from build123d import *

# Parameters (mm, degrees)
SKETCH1_W           = 50.8
SKETCH1_H           = 38.1
BOSS_EXTRUDE1_DEPTH = 19.05
SKETCH2_W           = 44.45
SKETCH2_H           = 31.75
CUT_EXTRUDE1_DEPTH  = 12.7
SKETCH3_R           = 4.7625
SKETCH3_R_2         = 2.38125
CUT_EXTRUDE2_DEPTH  = 42.639734629
SKETCH4_W           = 7.9375
SKETCH4_H           = 7.9375
BOSS_EXTRUDE2_DEPTH = 12.7
SKETCH5_R           = 1.778
CUT_EXTRUDE3_DEPTH  = 42.639734629


with BuildPart() as part:
    # Sketch1 → Boss-Extrude1 (new body)
    with BuildSketch(Plane.XY):
        with Locations((6.35, 0)):
            Rectangle(SKETCH1_W, SKETCH1_H)
    extrude(amount=-BOSS_EXTRUDE1_DEPTH)

    # Sketch2 → Cut-Extrude1 (cut)
    with BuildSketch(Plane(origin=(0, 0, -19.05), x_dir=(-1, 0, 0), z_dir=(0, 0, -1))):
        with Locations((-6.35, 0)):
            Rectangle(SKETCH2_W, SKETCH2_H)
    extrude(amount=-CUT_EXTRUDE1_DEPTH, mode=Mode.SUBTRACT)

    # Sketch3 → Cut-Extrude2 (cut, through all)
    with BuildSketch(Plane.XY):
        Circle(SKETCH3_R)
        with Locations((17.462302917, 0.082964446)):
            Circle(SKETCH3_R_2)
    extrude(amount=-CUT_EXTRUDE2_DEPTH, mode=Mode.SUBTRACT)

    # Sketch4 → Boss-Extrude2 (add)
    with BuildSketch(Plane(origin=(0, 0, -6.35), x_dir=(-1, 0, 0), z_dir=(0, 0, -1))):
        with Locations((-27.78125, 15.08125)):
            Rectangle(SKETCH4_W, SKETCH4_H)
        with Locations((15.08125, 15.08125)):
            Rectangle(SKETCH4_W, SKETCH4_H)
        with Locations((15.08125, -15.08125)):
            Rectangle(SKETCH4_W, SKETCH4_H)
        with Locations((-27.78125, -15.08125)):
            Rectangle(SKETCH4_W, SKETCH4_H)
    extrude(amount=BOSS_EXTRUDE2_DEPTH)

    # Sketch5 → Cut-Extrude3 (cut, through all)
    with BuildSketch(Plane(origin=(0, 0, -19.05), x_dir=(-1, 0, 0), z_dir=(0, 0, -1))):
        with Locations((-27.78125, 15.08125)):
            Circle(SKETCH5_R)
        with Locations((15.08125, 15.08125)):
            Circle(SKETCH5_R)
        with Locations((15.08125, -15.08125)):
            Circle(SKETCH5_R)
        with Locations((-27.78125, -15.08125)):
            Circle(SKETCH5_R)
    extrude(amount=-CUT_EXTRUDE3_DEPTH, mode=Mode.SUBTRACT)


solid = part.part
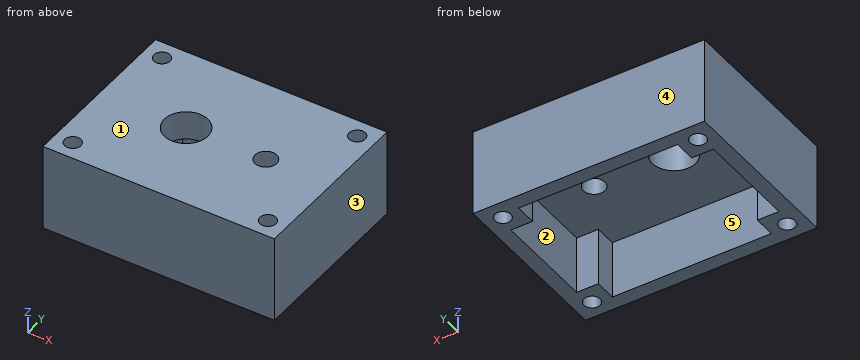
Geometry: final body of the model. Coordinates: model frame, mm. Face numbers are marked on the shaded views. A direction names the side the tool comes from. Give positions to 0.01 mm unless a question says otherwise; leave off trailing zeros. Order: outer loops, then holes, each group sorted by start corner. A loop starts at its lowest first (then second) coordinate and runs counter-clockwise, first axis right, second up. Notation, with made-up numbers: (-10, 43) -> (-6, 43) arc R36 ccw to (-6, 78) -> close; hole circle Ø9 at (81.25, -38). An arc over 180 degrees is marked (long way). Put each result on its own line as item: value.
Q1. Section C-C, the plane x = -15. Return loops of the section in (y, z).
Here are the results:
outline: (-19.05, -19.05) -> (-16.86, -19.05) -> (-16.86, 0) -> (-19.05, 0) -> close; (-13.31, -19.05) -> (-11.11, -19.05) -> (-11.11, -6.35) -> (11.11, -6.35) -> (11.11, -19.05) -> (13.31, -19.05) -> (13.31, 0) -> (-13.31, 0) -> close; (16.86, -19.05) -> (19.05, -19.05) -> (19.05, 0) -> (16.86, 0) -> close
Q2. Section B-B, the plane y = -9. Return loops of the section in (x, z) (3 decimals).
Here are the results:
outline: (-19.05, -19.05) -> (-15.875, -19.05) -> (-15.875, -6.35) -> (28.575, -6.35) -> (28.575, -19.05) -> (31.75, -19.05) -> (31.75, 0) -> (-19.05, 0) -> close
Q3. Reachability of the marked faces 1 and 2 from +Z, -Z, +X, -X, +Y, -Y: full face, straight path, thin tool, end or side. Return the list, or none.
Here are the results:
face 1: +Z, +X, -X, +Y, -Y
face 2: -Z
Q4. Section D-D, the plane z = -12.75. Count the separate pieces of the cut face and the enclosed holes in it, then the cut area to 3 significant figures.
Here are the results:
separate pieces: 1
enclosed holes: 5
area: 575 mm^2
Q5. Pin query (flat end, axial travel): pin 1 (5.5 mm diameter, centred on x = 17.46, y = 0.08, fed in from -Z); pin 2 (2 mm diameter, centred on x = 27.78, y = 15.08, fed in from +Z). Return the tip coordinate at first contact, or that it passes through.
Here are the results:
pin 1: stops at z = -6.35
pin 2: passes through
Q6. Draft query along X for the marked faces 3, 4 and 5. Return one class per face: released by +X, released by -X, zero draft, split by the parting line, or undercut.
Here are the results:
face 3: released by +X
face 4: zero draft
face 5: undercut
Q7. Material intervals for L1, parallel to Y at x = -15, z = -7; L2, parallel to X at y = -15, z = -12.25; L3, parallel to X at y = -5, z = -11 (3 decimals), sorted ascending.
Here are the results:
L1: y = -19.05 to -16.86, -13.31 to -11.11, 11.11 to 13.31, 16.86 to 19.05
L2: x = -19.05 to -16.86, -13.31 to -11.11, 23.81 to 26.01, 29.56 to 31.75
L3: x = -19.05 to -15.875, 28.575 to 31.75
